Build history of the part. All positions in model axes, mm. A direction names the side the tool comes from. Round coordinates to 2 decimals unless told otherwise and drop trailing zeros. Write each loop counter-clockwise with the first axis right and the second up, starting at its lowest first coordinate (ties: lowest second). Pieces come first, ordered by that corner, then holes.
Autodesk Inventor part; units mm, degrees
ref_plane "YZ Plane" through (0, 0, 0) normal (1, 0, 0) x (0, 1, 0)
ref_plane "XZ Plane" through (0, 0, 0) normal (0, 1, 0) x (-1, 0, 0)
ref_plane "XY Plane" through (0, 0, 0) normal (0, 0, 1) x (1, 0, 0)
sketch "Sketch1" plane through (0, 0, 0) normal (0, 1, 0) x (-1, 0, 0)
  line L0 (0, 0) -> (83.3, 0)
  line L1 (83.3, 0) -> (83.3, -124)
  line L2 (83.3, -124) -> (0, -124)
  line L3 (0, -124) -> (0, 0)
  dimension "d0" = 124
  dimension "d1" = 83.3
extrude "Lid Body" add sketch "Sketch1" along normal blind 4
fillet "4mm Fillet" radius 4 4 edges at (0, 2, -124) (-83.3, 2, -124) (-83.3, 2, 0) (0, 2, 0)
sketch "Sketch2" plane through (0, 4, 0) normal (0, 1, 0) x (1, 0, 0)
  circle A0 centre (-80.3, 3) radius 1.5
  line L0 (-83.3, 124) -> (-83.3, 0)
  line L1 (-83.3, 0) -> (0, 0)
  line L2 (-83.3, 62) -> (0, 62)
  line L3 (0, 0) -> (0, 124)
  line L4 (-41.65, 0) -> (-41.65, 124)
  circle A1 centre (-80.3, 121) radius 1.5
  circle A2 centre (-3, 3) radius 1.5
  circle A3 centre (-3, 121) radius 1.5
  dimension "d5" = 3
  dimension "d6" = 3
  dimension "d7" = 3
extrude "Extrusion2" cut sketch "Sketch2" against normal through all contours A0 | A1 | A2 | A3
sketch "Sketch3" plane through (0, 4, 0) normal (0, 1, 0) x (1, 0, 0)
  line L0 (-83.3, 0) -> (0, 0)
  line L1 (0, 0) -> (0, 124)
  line L2 (0, 124) -> (-83.3, 124)
  line L3 (-83.3, 124) -> (-83.3, 0)
  line L4 (-78.3, 5) -> (-5, 5)
  line L5 (-5, 5) -> (-5, 119)
  line L6 (-5, 119) -> (-78.3, 119)
  line L7 (-78.3, 119) -> (-78.3, 5)
  line L8 (-68.095, 22.786) -> (-14.795, 22.786)
  line L9 (-14.795, 22.786) -> (-14.795, 100.786)
  line L10 (-14.795, 100.786) -> (-68.095, 100.786)
  line L11 (-68.095, 100.786) -> (-68.095, 22.786)
  dimension "d11" = 5
  dimension "d12" = 53.3
  dimension "d13" = 78
  dimension "d14" = 10.205
  dimension "d15" = 17.786
extrude "Extrusion3" cut sketch "Sketch3" against normal through all contours L11 L10 L9 L8
fillet "2mm Fillet" [suppressed]
properties part number "LidTest01"
1) Pin check, flat tip, straight feed: pin 1 Ø3 at (x, z) = (-16.5, -93) entering from -Y. Stop position of the tip, or through.
Results:
pin 1: passes through
2) Wall check: L1, parallel to Z at x = -3, y = 2.05; L2, parallel to X at y = 2.35, z = -121; L3, parallel to X at y = 2.55, z = -48 (3 decimals). Give the ranges that are in metal, low to high.
Results:
L1: z = -123.87 to -122.5, -119.5 to -4.5, -1.5 to -0.13
L2: x = -83.17 to -81.8, -78.8 to -4.5, -1.5 to -0.13
L3: x = -83.3 to -68.095, -14.795 to 0
3) Slice it at A-A (x = -51.5). Write the cut outline in (y, z).
Results:
outline: (0, -124) - (4, -124) - (4, -100.79) - (0, -100.79) - close; (0, -22.79) - (4, -22.79) - (4, 0) - (0, 0) - close
4) Slice it at B-B (z = -96.5). Write the cut outline in (x, y) (3 decimals), plus the area to 3 significant figures.
Results:
outline: (-83.3, 0) - (-68.095, 0) - (-68.095, 4) - (-83.3, 4) - close; (-14.795, 0) - (0, 0) - (0, 4) - (-14.795, 4) - close
area: 120 mm2
5) Which spindle directions (+Z, -Z, +X, -X, +Y, -Y) get a long thin tool onto all of the face, cutting with end or side? Do faces 1 (the flat face through (-13, 0, -61)), 2 (the flat face through (-41, 2, -100.786)). Say none if no direction does.
Results:
face 1: +Z, -Z, +X, -X, -Y
face 2: +Y, -Y
6) Slice it at C-C (y = 1.9). Write the cut outline in (x, z) (3 decimals), plus the area to 3 significant figures.
Results:
outline: (-83.3, -120) arc R4 ccw to (-79.3, -124) - (-4, -124) arc R4 ccw to (0, -120) - (0, -4) arc R4 ccw to (-4, 0) - (-79.3, 0) arc R4 ccw to (-83.3, -4) - close; hole circle Ø3 at (-80.3, -121); hole circle Ø3 at (-80.3, -3); hole (-68.095, -100.786) - (-14.795, -100.786) - (-14.795, -22.786) - (-68.095, -22.786) - close; hole circle Ø3 at (-3, -121); hole circle Ø3 at (-3, -3)
area: 6,130 mm2
7) Mould opens along Z. For faces 3 (the flat face through (0, 2, -63)), 4 (the flat face through (-42, 2, -22.786)), 5 (the cylindrical face through (-82.159, 2.028, -1.203)) say: released by +Z, released by -Z, zero draft, split by the parting line, or undercut.
Results:
face 3: zero draft
face 4: undercut
face 5: released by +Z
